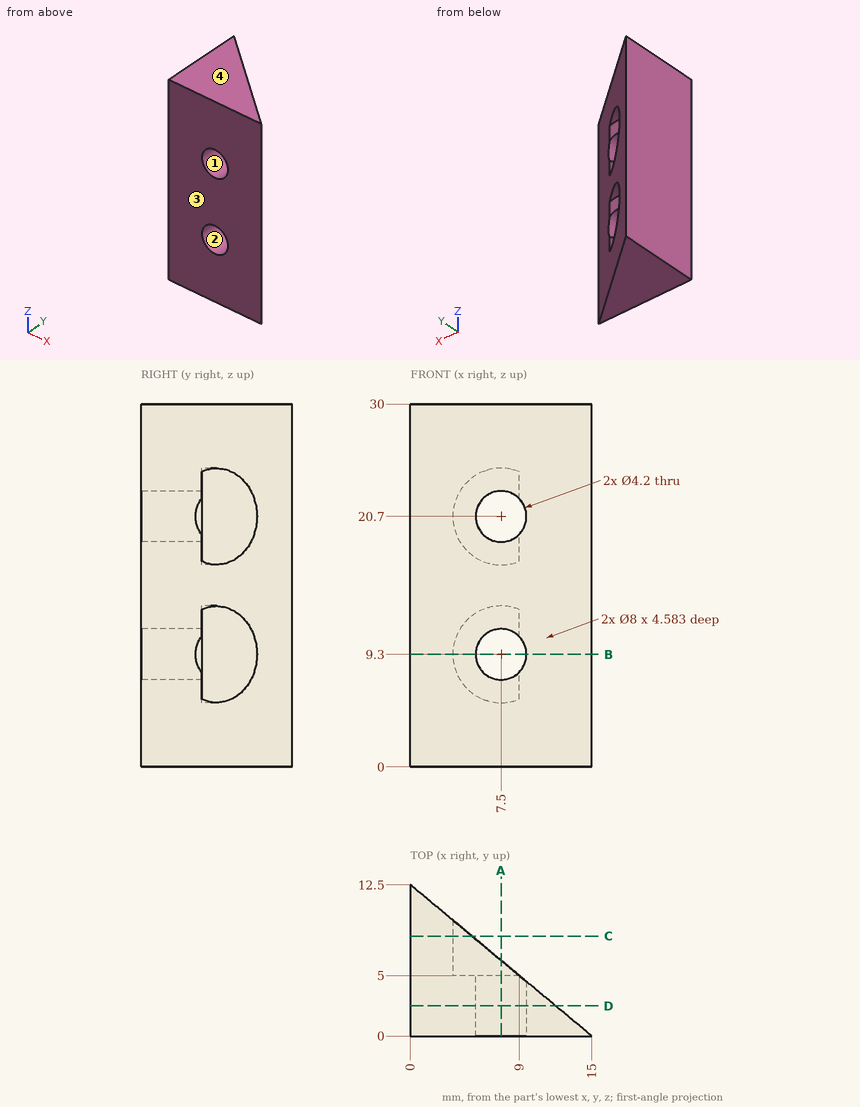
Verification items for this drawing (mm, ordinates from the low corner). Round coordinates to 2 decimals unless told otherwise and drop trailing zeros. Loops run counter-clockwise (first coordinate to the right, second up) from the corner with the lowest first, then second, coordinate; pieces in that order, holes last. Notation, with made-up numbers: (13.25, 21) -> (36.25, 21) arc R19 ccw to (36.25, 27) -> close; hole circle Ø10 at (-37.75, 54). An arc over 180 degrees is marked (long way). Write item = value, one per line. Start each with the question number.
1) Sectioned sample at D-D, the plane y = 2.5. Record the cut outline in (x, z).
2) Sectioned sample at B-B, the plane z = 9.3. Record the cut outline in (x, y).
3) Sectioned sample at A-A, the plane x = 7.5. Record the cut outline in (y, z).
4) Release check for a two-part mould opening along Z. For the marked faces 1, 2, 3 and 4 record: released by +Z, released by -Z, zero draft, split by the parting line, or undercut.
5) Sectioned sample at C-C, the plane y = 8.25. Record the cut outline in (x, z).
6) Thickness scan on probe 1 along Z at (x, y) = (7.5, 3.45); probe 2 along Z at (x, y) = (7.5, 6.2); probe 3 along X at (y, z) = (6.25, 9.3). Record the ranges inside material, lowest first.
7) Gauge pin test, flat ends, axial feed: pin 1 Ø9 at (x, z) = (7.5, 20.7) entering from +Y; pin 2 Ø4.5 at (x, z) = (5.5, 8) entering from +Y; pin 3 Ø3.5 at (x, z) = (7.5, 20.7) entering from -Y; pin 4 Ø6.5 at (x, z) = (7.5, 9.3) entering from +Y. Record the tip position at first contact, or that the pin passes through.
Results are:
q1.outline = (0, 0) -> (12, 0) -> (12, 30) -> (0, 30) -> close; hole circle Ø4.2 at (7.5, 9.3); hole circle Ø4.2 at (7.5, 20.7)
q2.outline = (0, 0) -> (5.4, 0) -> (5.4, 5) -> (3.5, 5) -> (3.5, 9.58) -> (0, 12.5) -> close; (9.6, 0) -> (15, 0) -> (9.6, 4.5) -> close
q3.outline = (0, 0) -> (6.25, 0) -> (6.25, 5.3) -> (5, 5.3) -> (5, 7.2) -> (0, 7.2) -> close; (0, 11.4) -> (5, 11.4) -> (5, 13.3) -> (6.25, 13.3) -> (6.25, 16.7) -> (5, 16.7) -> (5, 18.6) -> (0, 18.6) -> close; (0, 22.8) -> (5, 22.8) -> (5, 24.7) -> (6.25, 24.7) -> (6.25, 30) -> (0, 30) -> close
q4.face_1 = undercut
q4.face_2 = undercut
q4.face_3 = zero draft
q4.face_4 = released by +Z
q5.outline = (0, 0) -> (5.1, 0) -> (5.1, 6.1) arc R4 cw to (5.1, 12.5) -> (5.1, 17.5) arc R4 cw to (5.1, 23.9) -> (5.1, 30) -> (0, 30) -> close
q6.probe_1 = 0 to 7.2, 11.4 to 18.6, 22.8 to 30
q6.probe_2 = 0 to 5.3, 13.3 to 16.7, 24.7 to 30
q6.probe_3 = 0 to 3.5
q7.pin_1 = 10
q7.pin_2 = 9.79
q7.pin_3 = through
q7.pin_4 = 5
